from build123d import *

# Parameters (mm, degrees)
PAD127_DEPTH            = 10
FILLET002_R             = 8
POCKET105_DEPTH         = 12
BODY089_PLACEMENT_ANGLE = 270


with BuildPart() as part:
    # Sketch257 → Pad127 (new body, symmetric)
    with BuildSketch(Plane.YZ):
        Polygon((0, 13), (-148.59068, 0), (30, 0), (30, 13), align=None)
    extrude(amount=PAD127_DEPTH, both=True)

    # Fillet002
    fillet002_edges = [part.edges().sort_by_distance(p)[0] for p in [
        (10, 30, 6.5),
        (-10, 30, 6.5),
    ]]
    fillet(fillet002_edges, radius=FILLET002_R)

    # Sketch258 (on Face8 of Fillet002) → Pocket105 (cut)
    with BuildSketch(Plane(origin=(0, 0, 13), x_dir=(0, -1, 0), z_dir=(0, 0, 1))):
        with BuildLine():
            ThreePointArc((-15.70466, 8), (-23.70466, 0), (-15.70466, -8))
            Line((-15.70466, -8), (134.29534, -8))
            ThreePointArc((134.29534, -8), (142.29534, 0), (134.29534, 8))
            Line((-15.70466, 8), (134.29534, 8))
        make_face()
    extrude(amount=-POCKET105_DEPTH, mode=Mode.SUBTRACT)


with BuildPart() as part_1:
    # Body089 placement: moved
    add(part.part.moved(Location((173, -150, 39))).rotate(Axis((173, -150, 39), (0, 0, 1)), BODY089_PLACEMENT_ANGLE))


solid = part_1.part
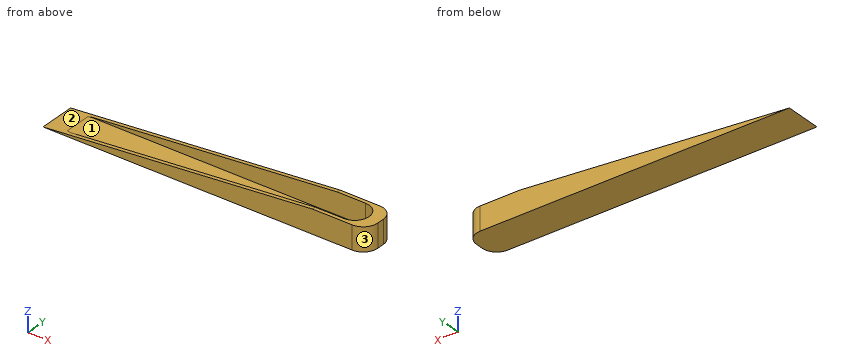
Here's how the part is built. I have some questions about the finished solid (model axes, mm). Face numbers are marked on the shaded views. Round coordinates to 2 decimals unless told otherwise and drop trailing zeros. Order: outer loops, then holes, each group sorted by start corner. A loop starts at its lowest first (then second) coordinate and runs counter-clockwise, first axis right, second up. Notation, with made-up numbers: M 27,89 L 37,89 A25 cw 37,123 Z; hole C 42.5,73.25 d10. An arc over 180 degrees is marked long. One line per question, with ' | ' between items.
1) I'm going to push flat-ended pins straight in: pin 1 Ø12 at (x, y) = (130, -142.5) entering from +Z; pin 2 Ø2 at (x, y) = (109.5, -156) entering from +Z; pin 3 Ø3 at (y, z) = (-157.5, 47.5) entering from +X; pin 4 Ø1.5 at (x, z) = (99, 46.5) entering from -Y. Where does each tip first touch, or does it pass through?
Checked values:
pin 1: stops at z = 48.76 | pin 2: stops at z = 40 | pin 3: stops at x = 201.93 | pin 4: passes through
2) Imagine slicing it at C-C, the plane z = 42. Write out the boundary of the cut face in (x, y).
Checked values:
outline: M 58.7,-160 L 195,-160 A8 ccw 203,-152 L 203,-148 A8 ccw 195,-140 L 58.7,-140 L 58.7,-142 L 188.7,-142 A8 cw 188.7,-158 L 58.7,-158 Z
3) We'd pull the mould along Y, two halves only. Please class the marked faces 1, 2 and 3: released by +Y, released by -Y, zero draft, split by the parting line, or undercut.
Checked values:
face 1: undercut | face 2: zero draft | face 3: released by -Y
4) Imagine slicing it at A-A, the plane x = 180.5. Write out the boundary of the cut face in (y, z).
Checked values:
outline: M -160,39 L -140,39 L -140,52 L -142,52 L -142,40 L -158,40 L -158,52 L -160,52 Z
5) Imagine slicing it at D-D, the plane x = 115. Write out the boundary of the cut face in (y, z), plus the area to 3 significant figures.
Checked values:
outline: M -160,39 L -140,39 L -140,46.93 L -142,46.93 L -142,40 L -158,40 L -158,46.93 L -160,46.93 Z | area: 47.7 mm²
6) Imagine slicing it at B-B, the plane y = -150. Write out the boundary of the cut face in (x, z), plus the area to 3 significant figures.
Checked values:
outline: M 24.41,39 L 203,39 L 203,52 L 196.7,52 L 196.7,40 L 35.84,40 Z | area: 248 mm²
7) I need wall thicknesses on line 1 (Y direction, x = 175.5, z = 50.25); line 2 (Z direction, x = 193, y = -153); line 3 (X direction, y = -150, z = 47.75). Which ranges of each line are inside material? Lowest first, please.
Checked values:
line 1: y = -160 to -158, -142 to -140 | line 2: z = 39 to 40 | line 3: x = 196.7 to 203
